Check sheet for the modelled part. Datum: model origin and axes. Units: mm. A direction names the side the tool comes from. Round coordinates to 2 decimals unless told otherwise and drop trailing zeros. Order: outer loops, then holes, each group sorted by start corner. A loop starts at its lowest first (then second) coordinate and runs counter-clockwise, first axis right, second up.
Q1. Depth check by flat-ended pin: P1, Ø5, axis at x = -14, y = 0, coming from the +Z side; P2, Ø3, axis at x = -6.5, z = 6, coming from the -Y side; P3, Ø3, axis at y = -18.5, z = 7.5, coming from the +X side. Enter the tip coordinate at first touch or a pass-through.
Q2. Set-up check for faces 1 (the flat face through (-29.506, -2.642, 4.437)), 2 (the flat face through (-16.78, 22.57, 4.44)), 3 (the flat face through (-10.315, 27.003, 4.437)), 4 (the flat face through (-11.631, 27.246, 4.437)), 5 (the flat face through (28.38, -5.378, 4.437)): record each of +Z, -Z, +X, -X, +Y, -Y from which the full face is reachable in a straight line by a thin tool's end or side.
Q3. Scan lines: probe 1 along Y at (x, z) = (0, 1.65); probe 2 along Y at (x, z) = (16, 4.5); probe 3 along X at (y, z) = (20, 7.5). Record each from-to range of solid material in increasing order.
Q4. Cross-section at A-A on x = 0. Record the cut outline in (y, z).
Q5. Mould release check, pull along Y, two halves, no side actions. Record for faces 6 (the flat face through (25.195, -12.496, 4.437)), 7 (the flat face through (22.73, -19, 4.44)), 8 (the flat face through (6.6, 28.88, 4.44)): +Y half, -Y half, draft (parallel to the pull), parting line (faces both ways), or undercut.
from build123d import *

# Parameters (mm, degrees)
PAD_DEPTH       = 9
SKETCH001_R     = 25
POCKET_DEPTH    = 7
SKETCH002_R     = 5
POCKET001_DEPTH = 2.001
SKETCH003_R     = 2
POCKET002_DEPTH = 2.001
SKETCH004_R     = 10
SKETCH004_R_2   = 5
PAD001_DEPTH    = 1


with BuildPart() as part:
    # Sketch → Pad (new body)
    with BuildSketch(Plane.XY):
        Polygon((-26.503024, 9.47509), (-27.894659, 10.03487), (-27.073648, 12.075934), (-25.682014, 11.516154), (-24.694497, 13.504422), (-25.98143, 14.27501), (-24.851234, 16.162511), (-23.564302, 15.391923), (-22.27791, 17.201231), (-23.428452, 18.163652), (-22.016901, 19.851113), (-20.866359, 18.888692), (-19.312767, 20.474488), (-20.298587, 21.605045), (-18.640438, 23.050915), (-17.654617, 21.920358), (-15.872079, 23.243596), (-16.668904, 24.514449), (-14.804986, 25.683127), (-14.00816, 24.412273), (-12.040568, 25.440369), (-12.628778, 26.820227), (-10.604979, 27.682919), (-10.016776, 26.303077), (-7.912578, 27.010715), (-8.277689, 28.465602), (-6.143855, 29.001097), (-5.778745, 27.546211), (-3.589754, 27.915968), (-3.722775, 29.410059), (-1.531443, 29.605156), (-1.398422, 28.111066), (0.821461, 28.133838), (0.923805, 29.630342), (3.118678, 29.480238), (3.016334, 27.983734), (5.21245, 27.658959), (5.547638, 29.121029), (7.692007, 28.629419), (7.356819, 27.167349), (9.47509, 26.503024), (10.03487, 27.894659), (12.075934, 27.073648), (11.516154, 25.682014), (13.504422, 24.694497), (14.27501, 25.98143), (16.162511, 24.851234), (15.391923, 23.564302), (17.201231, 22.27791), (18.163652, 23.428452), (19.851113, 22.016901), (18.888692, 20.866359), (20.474488, 19.312767), (21.605045, 20.298587), (23.050915, 18.640438), (21.920358, 17.654617), (23.243596, 15.872079), (24.514448, 16.668904), (25.683127, 14.804986), (24.412273, 14.00816), (25.440369, 12.040568), (26.820227, 12.628778), (27.682935, 10.604985), (26.303077, 10.016776), (27.010715, 7.912578), (28.465602, 8.277689), (29.001097, 6.143855), (27.546211, 5.778745), (27.915968, 3.589754), (29.410059, 3.722775), (29.605156, 1.531443), (28.111066, 1.398422), (28.133838, -0.821461), (29.630342, -0.923805), (29.480238, -3.118678), (27.983734, -3.016334), (27.658959, -5.21245), (29.121029, -5.547638), (28.629419, -7.692007), (27.167349, -7.356819), (26.503024, -9.47509), (27.894659, -10.03487), (27.073648, -12.075934), (25.682014, -11.516154), (24.694497, -13.504422), (25.98143, -14.27501), (24.851235, -16.162511), (23.564302, -15.391923), (22.27791, -17.201231), (23.428452, -18.163652), (22.016901, -19.851113), (20.866359, -18.888692), (19.312767, -20.474488), (20.298587, -21.605045), (18.640438, -23.050915), (17.654617, -21.920358), (15.872079, -23.243596), (16.668904, -24.514449), (14.804986, -25.683127), (14.00816, -24.412273), (12.040568, -25.440369), (12.628778, -26.820227), (10.604986, -27.682935), (10.016776, -26.303077), (7.912578, -27.010715), (8.277689, -28.465602), (6.143855, -29.001097), (5.778745, -27.546211), (3.589754, -27.915968), (3.722775, -29.410059), (1.531443, -29.605156), (1.398422, -28.111066), (-0.821461, -28.133838), (-0.923805, -29.630342), (-3.118678, -29.480238), (-3.016334, -27.983734), (-5.21245, -27.658959), (-5.547638, -29.121029), (-7.692007, -28.629419), (-7.356819, -27.167349), (-9.47509, -26.503024), (-10.03487, -27.894659), (-12.075934, -27.073648), (-11.516154, -25.682014), (-13.504422, -24.694497), (-14.27501, -25.98143), (-16.162511, -24.851234), (-15.391923, -23.564302), (-17.201231, -22.27791), (-18.163652, -23.428452), (-19.851113, -22.016901), (-18.888692, -20.866359), (-20.474488, -19.312767), (-21.605045, -20.298587), (-23.050915, -18.640438), (-21.920358, -17.654617), (-23.243596, -15.872079), (-24.514449, -16.668904), (-25.683127, -14.804986), (-24.412273, -14.00816), (-25.440369, -12.040568), (-26.820227, -12.628778), (-27.682935, -10.604985), (-26.303077, -10.016776), (-27.010715, -7.912578), (-28.465602, -8.277689), (-29.001097, -6.143855), (-27.546211, -5.778745), (-27.915968, -3.589754), (-29.410059, -3.722775), (-29.605156, -1.531443), (-28.111066, -1.398422), (-28.133838, 0.821461), (-29.630342, 0.923805), (-29.480238, 3.118678), (-27.983734, 3.016334), (-27.658959, 5.21245), (-29.121029, 5.547638), (-28.629419, 7.692007), (-27.167349, 7.356819), align=None)
    extrude(amount=PAD_DEPTH)

    # Sketch001 (on Face162 of Pad) → Pocket (cut)
    with BuildSketch(Plane.XY.offset(9)):
        Circle(SKETCH001_R)
    extrude(amount=-POCKET_DEPTH, mode=Mode.SUBTRACT)

    # Sketch002 (on Face164 of Pocket) → Pocket001 (cut, through all)
    with BuildSketch(Plane.XY.offset(2)):
        Circle(SKETCH002_R)
    extrude(amount=-POCKET001_DEPTH, mode=Mode.SUBTRACT)

    # Sketch003 (on Face165 of Pocket001) → Pocket002 (cut, through all)
    with BuildSketch(Plane.XY.offset(2)):
        with Locations((0, 14)):
            Circle(SKETCH003_R)
        with Locations((14, 0)):
            Circle(SKETCH003_R)
        with Locations((0, -14)):
            Circle(SKETCH003_R)
        with Locations((-14, 0)):
            Circle(SKETCH003_R)
    extrude(amount=-POCKET002_DEPTH, mode=Mode.SUBTRACT)

    # Sketch004 (on Face169 of Pocket002) → Pad001 (join)
    with BuildSketch(Plane.XY.offset(2)):
        Circle(SKETCH004_R)
        Circle(SKETCH004_R_2, mode=Mode.SUBTRACT)
    extrude(amount=PAD001_DEPTH)


solid = part.part
Results found:
1. P1: stops at z = 2
1. P2: stops at y = -29.12
1. P3: stops at x = 23.43
2. face 1: +Z, -Z, -X, -Y
2. face 2: +Z, -Z
2. face 3: +Z, -Z, +Y
2. face 4: +Z, -Z, -X, +Y
2. face 5: +Z, -Z, +X
3. probe 1: y = -28.13 to -16, -12 to -5, 5 to 12, 16 to 28.13
3. probe 2: y = -24.93 to -23.45, -23.15 to -19.21, 19.21 to 23.13, 24.58 to 24.95
3. probe 3: x = -19.78 to -15, 15 to 19.77, 21.26 to 21.87
4. outline: (-28.13, 0) - (-16, 0) - (-16, 2) - (-25, 2) - (-25, 9) - (-28.13, 9) - close; (-12, 0) - (-5, 0) - (-5, 3) - (-10, 3) - (-10, 2) - (-12, 2) - close; (5, 0) - (12, 0) - (12, 2) - (10, 2) - (10, 3) - (5, 3) - close; (16, 0) - (28.13, 0) - (28.13, 9) - (25, 9) - (25, 2) - (16, 2) - close
5. face 6: undercut
5. face 7: -Y half
5. face 8: +Y half
